Can you work these out from the model? Positions are in its coordinate system, mm. Face numbers are marked on the shaded views. A direction names the side the tool comes from. Give positions to 0.01 mm unless a question says otherwise; leave off trailing zeros. Order: outer loops, then holes, each group sorted by start corner. A loop starts at its lowest first (then second) coordinate and runs counter-clockwise, first axis right, second up. Notation, with made-up numbers: (19, -23.5) -> (23, -23.5) arc R25 cw to (23, 3.5) -> close; hole circle Ø8 at (-33.75, 44). An arc over 180 degrees is marked (long way). Answer as a JSON object with one key per item and string values.
Autodesk Inventor part; units mm, degrees
ref_plane "YZ Plane" through (0, 0, 0) normal (1, 0, 0) x (0, 1, 0)
ref_plane "XZ Plane" through (0, 0, 0) normal (0, 1, 0) x (-1, 0, 0)
ref_plane "XY Plane" through (0, 0, 0) normal (0, 0, 1) x (1, 0, 0)
sketch "Boceto1" plane through (0, 0, 0) normal (0, 1, 0) x (-1, 0, 0)
  line L0 (0, 0) -> (17, 0)
  line L1 (17, 0) -> (17, -17)
  line L2 (17, -17) -> (0, -17)
  line L3 (0, -17) -> (0, 0)
  circle A0 centre (17, 0) radius 1.5
  circle A1 centre (17, -17) radius 1.5
  circle A2 centre (0, -17) radius 1.5
  circle A3 centre (0, 0) radius 1.5
  circle A4 centre (8.5, -8.5) radius 14.1421
  dimension "d0" = 17
  dimension "d1" = 17
  dimension "d2" = 3
  dimension "d3" = 3
  dimension "d4" = 3
  dimension "d5" = 3
extrude "Extrusión1" add sketch "Boceto1" along normal blind 2 contours L0 A0 L1 A1 L2 A2 L3 A3 | A4
sketch "Boceto2" plane through (-8.5, 2, -8.5) normal (0, 1, 0) x (1, 0, 0)
  circle A0 centre (8.5, -8.5) radius 1.5
  circle A1 centre (8.5, 8.5) radius 1.5
  circle A2 centre (8.5, 8.5) radius 1.5
  circle A3 centre (-8.5, 8.5) radius 1.5
  circle A4 centre (-8.5, 8.5) radius 1.5
  circle A5 centre (-8.5, -8.5) radius 1.5
  circle A6 centre (-8.5, -8.5) radius 1.5
extrude "Extrusión2" add sketch "Boceto2" against normal blind 4
sketch "Boceto3" plane through (-8.5, 0, -8.5) normal (0, -1, 0) x (1, 0, 0)
  circle A0 centre (0, 0) radius 6.5
  point P0 (8.5, 8.5)
  dimension "d10" = 13
extrude "Extrusión3" add sketch "Boceto3" along normal blind 15
sketch "Boceto4" plane through (-8.5, 0, -8.5) normal (0, -1, 0) x (1, 0, 0)
  circle A0 centre (0, 0) radius 6.5
  circle A1 centre (0, 0) radius 13.6366
  circle A2 centre (0, 0) radius 6.5
  circle A3 centre (0, 0) radius 14.1421
  point P0 (8.5, 8.5)
extrude "Extrusión4" cut sketch "Boceto4" against normal blind 10 contours A3
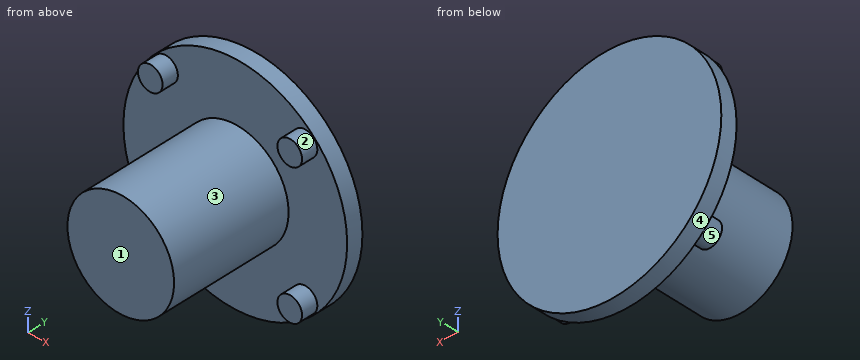
1. For the marked faces 4 and 5, which set-ups out of +Z, -Z, +X, -X, +Y, -Y let a thin tool reach every point of the face, with its end or its side?
Worked answers:
{"face 4": "+Y, -Y", "face 5": "-Y"}
2. If we section it at D-D on z = -17: Please give me the cut outline in (x, y).
Worked answers:
{"outline": "(-19.16, 0) -> (-18.5, 0) -> (-18.5, -2) -> (-15.5, -2) -> (-15.5, 0) -> (-1.5, 0) -> (-1.5, -2) -> (1.5, -2) -> (1.5, 0) -> (2.16, 0) -> (2.16, 2) -> (-19.16, 2) -> close"}
3. Please list where these lines run through material, in increasing order: L1, parallel to Y at x = -13.25, z = -4; L2, parallel to Z at x = -9.5, y = -13; L3, parallel to X at y = -9.5, z = -2.5.
Worked answers:
{"L1": "0 to 2", "L2": "-14.92 to -2.08", "L3": "-11 to -6"}
4. Will these pins go through, and if not, where does the flat tip stop? pin 1 Ø4 at (y, z) = (-6.5, -15) entering from -X; pin 2 Ø0.9 at (x, z) = (-16.5, -17.5) entering from -Y; pin 3 Ø6 at (x, y) = (-11.5, -6) entering from +Z; pin 4 Ø5 at (x, z) = (-16.5, -9) entering from -Y.
Worked answers:
{"pin 1": "x = -13.19", "pin 2": "y = -2", "pin 3": "z = -2", "pin 4": "y = -15"}
5. If we mould it in two halves opening along Z, with no side actions, what happens to the marked faces 1, 2 and 3? For each: +Z half, -Z half, draft (parallel to the pull), parting line (faces both ways), or undercut.
Worked answers:
{"face 1": "draft", "face 2": "undercut", "face 3": "parting line"}
6. If we section it at A-A on z = -9: Please give me the cut outline in (x, y).
Worked answers:
{"outline": "(-22.13, 0) -> (-14.98, 0) -> (-14.98, -15) -> (-2.02, -15) -> (-2.02, 0) -> (5.13, 0) -> (5.13, 2) -> (-22.13, 2) -> close"}
7. If we section it at C-C on y = -10: Please give me the cut outline in (x, z).
Worked answers:
{"outline": "circle Ø13 at (-8.5, -8.5)"}
8. If we section it at B-B on x = -10: Please give me the cut outline in (y, z), then the cut area to 3 significant figures.
Worked answers:
{"outline": "(-15, -14.82) -> (0, -14.82) -> (0, -22.05) -> (2, -22.05) -> (2, 5.05) -> (0, 5.05) -> (0, -2.18) -> (-15, -2.18) -> close", "area": "244 mm²"}
